```python
from build123d import *

# Parameters (mm, degrees)
SKETCH2_R           = 2.88
BOSS_EXTRUDE1_DEPTH = 0.250717968
SKETCH3_R           = 2.88
BOSS_EXTRUDE2_DEPTH = 0.069282032
BOSS_EXTRUDE2_TAPER = -59.999999992
SKETCH4_R           = 3
BOSS_EXTRUDE3_DEPTH = 29.68
SKETCH5_R           = 1.5705
BOSS_EXTRUDE4_DEPTH = 0.875
SKETCH6_R           = 1.5705
BOSS_EXTRUDE5_DEPTH = 0.4295
BOSS_EXTRUDE5_TAPER = -45
SKETCH7_R           = 2
BOSS_EXTRUDE6_DEPTH = 5.6955
CUT_EXTRUDE1_DEPTH  = 2
CHAMFER1_SIZE       = 0.4295
FILLET1_R           = 0.195


with BuildPart() as part:
    # Sketch1 → Revolve1 (revolve)
    with BuildSketch(Plane(origin=(0, 0, 0), x_dir=(-1, 0, 0), z_dir=(0, 0, -1))):
        with BuildLine():
            Line((0, 4.5), (0, 0))
            Line((0, 0), (4, 0))
            Line((4, 0), (4, 4.5))
            Line((4, 4.5), (2.2, 4.5))
            ThreePointArc((2.2, 4.5), (2, 4.3), (1.8, 4.5))
            Line((1.8, 4.5), (0, 4.5))
        make_face()
    revolve(axis=Axis((0, 0, 0), (-1, 0, 0)))

    # Sketch2 → Boss-Extrude1 (add)
    with BuildSketch(Plane(origin=(0, 0, 0), x_dir=(0, 0, -1), z_dir=(1, 0, 0))):
        Circle(SKETCH2_R)
    extrude(amount=BOSS_EXTRUDE1_DEPTH)

    # Sketch3 → Boss-Extrude2 (add)
    with BuildSketch(Plane(origin=(0.250717968, 0, 0), x_dir=(0, 0, -1), z_dir=(1, 0, 0))):
        Circle(SKETCH3_R)
    extrude(amount=BOSS_EXTRUDE2_DEPTH, taper=BOSS_EXTRUDE2_TAPER)

    # Sketch4 → Boss-Extrude3 (add)
    with BuildSketch(Plane(origin=(0.32, 0, 0), x_dir=(0, 0, -1), z_dir=(1, 0, 0))):
        Circle(SKETCH4_R)
    extrude(amount=BOSS_EXTRUDE3_DEPTH)

    # Sketch5 → Boss-Extrude4 (add)
    with BuildSketch(Plane(origin=(30, 0, 0), x_dir=(0, 0, -1), z_dir=(1, 0, 0))):
        Circle(SKETCH5_R)
    extrude(amount=BOSS_EXTRUDE4_DEPTH)

    # Sketch6 → Boss-Extrude5 (add)
    with BuildSketch(Plane(origin=(30.875, 0, 0), x_dir=(0, 0, -1), z_dir=(1, 0, 0))):
        Circle(SKETCH6_R)
    extrude(amount=BOSS_EXTRUDE5_DEPTH, taper=BOSS_EXTRUDE5_TAPER)

    # Sketch7 → Boss-Extrude6 (add)
    with BuildSketch(Plane(origin=(31.3045, 0, 0), x_dir=(0, 0, -1), z_dir=(1, 0, 0))):
        Circle(SKETCH7_R)
    extrude(amount=BOSS_EXTRUDE6_DEPTH)

    # Sketch8 → Cut-Extrude1 (cut)
    with BuildSketch(Plane.ZY.offset(4)):
        Polygon((1.5, -0.866025404), (1.5, 0.866025404), (0, 1.732050808), (-1.5, 0.866025404), (-1.5, -0.866025404), (0, -1.732050808), align=None)
    extrude(amount=-CUT_EXTRUDE1_DEPTH, mode=Mode.SUBTRACT)

    # Sketch9 → Cut-Revolve1 (revolve, cut)
    with BuildSketch(Plane.XY):
        Polygon((-2, 1.44), (-2, 0), (-1.168615612, 0), align=None)
    revolve(axis=Axis((-2, 0, 0), (1, 0, 0)), mode=Mode.SUBTRACT)

    # Chamfer1
    chamfer1_edges = [part.edges().sort_by_distance(p)[0] for p in [
        (37, 0, 2),
        (-4, -4.5, 0),
    ]]
    chamfer(chamfer1_edges, length=CHAMFER1_SIZE)

    # Fillet1
    fillet1_edges = [part.edges().sort_by_distance(p)[0] for p in [
        (0, 0, 2.88),
    ]]
    fillet(fillet1_edges, radius=FILLET1_R)


solid = part.part
```
Check sheet for the modelled part. Datum: model origin and axes. Units: mm. A direction names the side the tool comes from. Give positions to 0.01 mm unless a question says otherwise; leave off trailing zeros. Write each loop counter-clockwise with the first axis right and the second up, starting at its lowest first coordinate (ties: lowest second). Pieces come first, ordered by that corner, then holes. Notation, with made-up numbers: (-36, 61) - (2, 61) arc R19 ccw to (2, 91) - close; hole circle Ø11 at (-28.5, -19.75). An arc over 180 degrees is marked (long way). Answer as a JSON object with one key per item and string values. Group by question number.
1) Access from +Z, -Z, +X, -X, +Y, -Y to the whole of each face (thin tool, end or side, straight path). Record for faces 4 (the face through (30, -1.3, -1.3)), 5 (the face through (-3.014, 1.293, 0.76)), 6 (the face through (34, -2, 0)).
2) Thickness scan on probe 1 along X at (y, z) = (-0.5, 2); probe 2 along X at (y, z) = (1.5, 2.75); probe 3 along X at (y, z) = (-0.5, -1.75). Record the ranges inside material, lowest first. Write a range as from..to.
3) Sectioned sample at A-A (x = 30.5). Record the cut outline in (y, z), then the cut area to 3 significant figures.
4) Release check for a two-part mould opening along Z. For faces 1 (the face through (-3, 0, -1.5)), 2 (the face through (-0.89, -0.59, -4.46)), 3 (the face through (0, 2, 3)) record: pulls with the +Z half, pulls with the -Z half, needs draft (parallel to the pull), parting line crosses it, or undercut.
5) Sectioned sample at B-B (x = 25). Record the cut outline in (y, z).
6) Depth check by flat-ended pin: P1, Ø2, axis at x = 30.5, y = 0, coming from the +Z side; P2, Ø4, axis at x = 14.5, y = -3, coming from the +Z side; P3, Ø3, axis at x = 31, y = 3.5, coming from the -Z side. Enter the tip coordinate at first touch or a pass-through.
Geometry results:
{
 "1": {"face 4": "none", "face 5": "-X", "face 6": "+X"},
 "2": {"probe 1": "x = -4..30", "probe 2": "x = -4..0", "probe 3": "x = -4..30, 31.12..36.75"},
 "3": {"outline": "circle Ø3.14 at (0, 0)", "area": "7.75 mm^2"},
 "4": {"face 1": "undercut", "face 2": "parting line crosses it", "face 3": "needs draft"},
 "5": {"outline": "circle Ø6 at (0, 0)"},
 "6": {"P1": "stops at z = 3", "P2": "stops at z = 2.83", "P3": "stops at z = -1.82"}
}
